Part model, mm, in its own coordinate system. A direction names the side the tool comes from. Give positions to 0.01 mm unless a question says otherwise; leave off trailing zeros. Loops run counter-clockwise (first coordinate to the right, second up) from the corner with the lowest first, then second, coordinate; pieces in that order, holes last. Notation, with made-up numbers: M -6.5,59.25 L 29.5,59.25 A18 ccw 29.5,91.25 Z; hole C -1,-35 d3. An arc over 180 degrees is marked long. Answer in a Markdown table with one row per item.
from build123d import *


# Not quite as in the source:
# - a fillet or chamfer that OpenCascade refuses, or shapes differently, is made with other operations: its cross-section is extruded or revolved along the edge and cut away or added


with BuildPart() as f1:
    # F0 (on Front) → F1 (revolve)
    with BuildSketch(Plane.XZ):
        Polygon((-35.814, 0), (0, 0), (0, 10.3124), (-1.905, 10.3124), (-1.905, 6.8072), (-5.8674, 6.8072), (-5.8674, 10.3124), (-7.8486, 10.3124), (-7.8486, 3.9243), (-9.7536, 3.9243), (-9.7536, 4.7625), (-35.814, 4.7625), align=None)
    revolve(axis=Axis((-27.8073139489, 0, 0), (-1, 0, 0)))

    # F2: fillet of radius 0.9398 on 2 edges, made by hand

    # F2_s1 → F2_t2 (revolve)
    with BuildSketch(Plane.XZ):
        with BuildLine():
            ThreePointArc((-7.8486, 4.8641), (-8.123861047, 4.199561047), (-8.7884, 3.9243))
            Line((-8.7884, 3.9243), (-7.8486, 3.9243))
            Line((-7.8486, 3.9243), (-7.8486, 4.8641))
        make_face()
    revolve(axis=Axis((-7.8486, 0, 0), (-1, 0, 0)))

    # F2_s3 → F2_t4 (revolve)
    with BuildSketch(Plane.XZ):
        with BuildLine():
            ThreePointArc((-8.8193080328, 3.9243), (-9.4468988071, 4.1645616808), (-9.7536, 4.7625))
            Line((-9.7536, 4.7625), (-9.7536, 3.9243))
            Line((-9.7536, 3.9243), (-8.8193080328, 3.9243))
        make_face()
    revolve(axis=Axis((-9.7536, 0, 0), (-1, 0, 0)))


solid = f1.part
(1) Saw through at C-C (z = -7.25). Write the cut outline in (x, y) (3 decimals), plus the area to 3 significant figures.
Recorded:
| item | result |
|---|---|
| outline | M -7.849,-7.334 L -5.867,-7.334 L -5.867,7.334 L -7.849,7.334 Z; M -1.905,-7.334 L 0,-7.334 L 0,7.334 L -1.905,7.334 Z |
| area | 57.0 mm^2 |
(2) Saw through at D-D (y = 8.75). Write the cut outline in (x, z) (3 decimals), plus the area to 3 significant figures.
Recorded:
| item | result |
|---|---|
| outline | M -7.849,-5.457 L -5.867,-5.457 L -5.867,5.457 L -7.849,5.457 Z; M -1.905,-5.457 L 0,-5.457 L 0,5.457 L -1.905,5.457 Z |
| area | 42.4 mm^2 |
(3) Pull direction X, two halves, no side cores. Call faces 1 (the face through (-35.814, 0, 0)), 2 (the face through (0, 0, 0)), 3 (the face through (-1.905, -2, 7)): +X half, -X half, draft (parallel to the pull), parting line (faces both ways), or undercut.
Recorded:
| item | result |
|---|---|
| face 1 | -X half |
| face 2 | +X half |
| face 3 | undercut |
(4) Drill centre lines: line 1 along X through (y, z) = (-3, 8.75) (3 decimals); line 2 along Y through (x, z) = (-19, -0.25); line 3 along X through (y, z) = (4, -5). Where is each one in solid material? Low to high.
Recorded:
| item | result |
|---|---|
| line 1 | x = -7.849 to -5.867, -1.905 to 0 |
| line 2 | y = -4.76 to 4.76 |
| line 3 | x = -7.85 to 0 |
(5) Pin check, flat tips, straight feed: pin 1 Ø5 at (x, y) = (-21, -2) entering from -Z; pin 2 Ø12 at (x, y) = (-26.5, -3.5) entering from +Z; pin 3 Ø6 at (x, z) = (-31, -4) entering from +Y. Stop position of each tip, or through.
Recorded:
| item | result |
|---|---|
| pin 1 | stops at z = -4.76 |
| pin 2 | stops at z = 4.76 |
| pin 3 | stops at y = 4.66 |
(6) Which spindle directions (+Z, -Z, +X, -X, +Y, -Y) get a long thin tool onto all of the face, cutting with end or side? Do faces 4 (the face through (-6.87, 8.7, 5.54)), 5 (the face through (-7.849, 2.44, 4.44)), 6 (the face through (-5.867, -2, -7)). Say none if no direction does.
Recorded:
| item | result |
|---|---|
| face 4 | +X, -X |
| face 5 | -X |
| face 6 | none |
